```python
from build123d import *

# Parameters (mm, degrees)
SKETCH1_R           = 38.1
BOSS_EXTRUDE1_DEPTH = 3.175
SKETCH2_W           = 38.1
SKETCH2_H           = 38.1
BOSS_EXTRUDE3_DEPTH = 76.2
CUT_EXTRUDE1_DEPTH  = 105.967247868
SKETCH6_R           = 1.4605
CUT_EXTRUDE2_DEPTH  = 105.967247868


with BuildPart() as part:
    # Sketch1 → Boss-Extrude1 (new body)
    with BuildSketch(Plane(origin=(0, 0, 0), x_dir=(1, 0, 0), z_dir=(0, 1, 0))):
        with Locations(Location((0, 0, 0), (0, 0, 270))):
            Circle(SKETCH1_R)
    extrude(amount=BOSS_EXTRUDE1_DEPTH)

    # Sketch2 → Boss-Extrude3 (add)
    with BuildSketch(Plane(origin=(0, 3.175, 0), x_dir=(1, 0, 0), z_dir=(0, 1, 0))):
        Rectangle(SKETCH2_W, SKETCH2_H)
    extrude(amount=BOSS_EXTRUDE3_DEPTH)

    # Sketch5 → Cut-Extrude1 (cut, through all)
    with BuildSketch(Plane.ZY.offset(19.05)):
        Polygon((0, 79.375), (-1.5875, 79.375), (-1.5875, 15.875), (1.5875, 15.875), (1.5875, 79.375), align=None)
    extrude(amount=-CUT_EXTRUDE1_DEPTH, mode=Mode.SUBTRACT)

    # Sketch6 → Cut-Extrude2 (cut, through all)
    with BuildSketch(Plane.XY.offset(19.05)):
        with Locations((0, 69.85)):
            Circle(SKETCH6_R)
    extrude(amount=-CUT_EXTRUDE2_DEPTH, mode=Mode.SUBTRACT)


solid = part.part
```
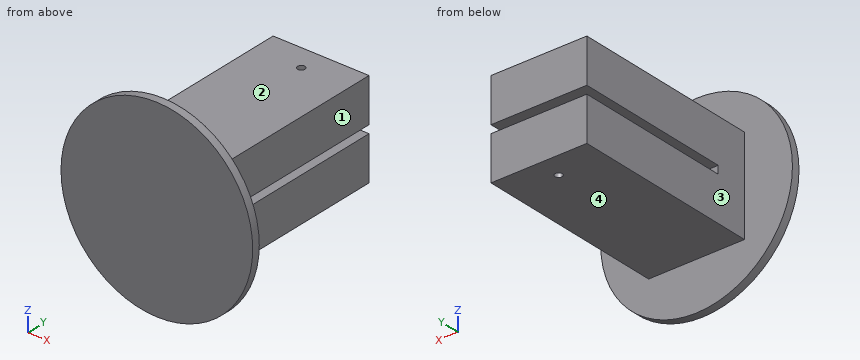
The model under review builds one solid part; all positions refer to its coordinate system, in mm. Face numbers are marked on the shaded views. A direction names the side the tool comes from. Round coordinates to 2 decimals unless told otherwise and drop trailing zeros. Loops run counter-clockwise (first coordinate to the right, second up) from the corner with the lowest first, then second, coordinate; pieces in that order, holes last.
1) Consider section C-C on y = 69.85. State the section outline as (x, z) points.
Values follow:
outline: (-19.05, -19.05) - (-1.46, -19.05) - (-1.46, -1.59) - (-19.05, -1.59) - close; (-19.05, 1.59) - (-1.46, 1.59) - (-1.46, 19.05) - (-19.05, 19.05) - close; (1.46, -19.05) - (19.05, -19.05) - (19.05, -1.59) - (1.46, -1.59) - close; (1.46, 1.59) - (19.05, 1.59) - (19.05, 19.05) - (1.46, 19.05) - close
2) Clearance check with flat-ended pins moving along their axes: P1, Ø1.5, axis at x = -28.5, z = -16.5, coming from the +Y side (3 decimals); P2, Ø19, axis at y = 39, z = -6.5, coming from the -X side; P3, Ø19, axis at x = 2, y = 27, coming from the -Z side. State where each tip first meets the part, or that it passes through.
Values follow:
P1: stops at y = 3.175
P2: stops at x = -19.05
P3: stops at z = -19.05
3) Consider section B-B on x = 0. Give the number of separate pieces and of enclosed holes in the cut face, then the cut area to 3 significant figures.
Values follow:
separate pieces: 3
enclosed holes: 0
area: 2,840 mm2
4) Wall thickness on line 1 along Z through (x, y) = (0, 24.5); line 2 along Y through (x, z) = (0, -9) (1 decimal); line 3 along X through (y, z) = (69.85, -7): over which ranges is each line inside the solid? List them lowest first.
Values follow:
line 1: z = -19.05 to -1.59, 1.59 to 19.05
line 2: y = 0 to 68.4, 71.3 to 79.4
line 3: x = -19.05 to -1.46, 1.46 to 19.05
5) Tool access review of the marked faces 1, 2, 3 and 4: name each direction out of +Z, -Z, +X, -X, +Y, -Y from which nothing blocks a thin tool from reaching the whole face with its end or side.
Values follow:
face 1: +Z, -Z, +X, +Y
face 2: +Z, +X, -X, +Y
face 3: +Z, -Z, -X, +Y
face 4: -Z, +X, -X, +Y
6) Consider section A-A on y = 20. State the section outline as (x, z) points.
Values follow:
outline: (-19.05, -19.05) - (19.05, -19.05) - (19.05, -1.59) - (-19.05, -1.59) - close; (-19.05, 1.59) - (19.05, 1.59) - (19.05, 19.05) - (-19.05, 19.05) - close
